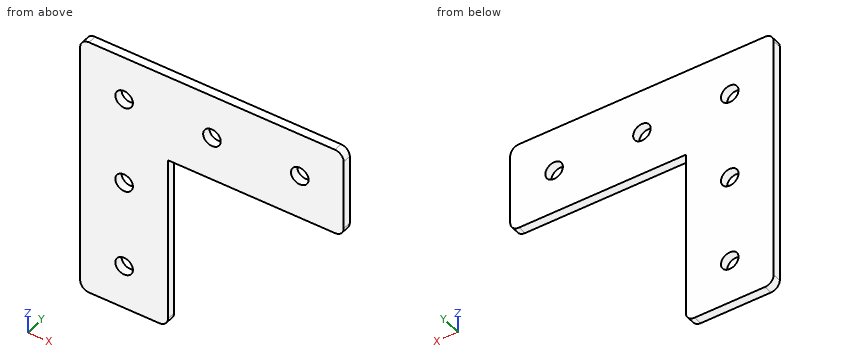
```python
from build123d import *

# Parameters (mm, degrees)
SKETCH1_R           = 2.54
BOSS_EXTRUDE1_DEPTH = 2.54
FILLET1_R           = 2.54


with BuildPart() as part:
    # Sketch1 → Boss-Extrude1 (new body)
    with BuildSketch(Plane(origin=(0, 0, 0), x_dir=(1, 0, 0), z_dir=(0, 1, 0))):
        Polygon((25.4, 76.2), (25.4, 25.4), (76.2, 25.4), (76.2, 0), (0, 0), (0, 76.2), align=None)
        with Locations((12.7, 12.7)):
            Circle(SKETCH1_R, mode=Mode.SUBTRACT)
        with Locations((38.1, 12.7)):
            Circle(SKETCH1_R, mode=Mode.SUBTRACT)
        with Locations((63.5, 12.7)):
            Circle(SKETCH1_R, mode=Mode.SUBTRACT)
        with Locations((12.7, 38.1)):
            Circle(SKETCH1_R, mode=Mode.SUBTRACT)
        with Locations((12.7, 63.5)):
            Circle(SKETCH1_R, mode=Mode.SUBTRACT)
    extrude(amount=BOSS_EXTRUDE1_DEPTH)

    # Fillet1
    fillet1_edges = [part.edges().sort_by_distance(p)[0] for p in [
        (0, 1.27, -76.2),
        (25.4, 1.27, -76.2),
        (76.2, 1.27, -25.4),
        (76.2, 1.27, 0),
        (0, 1.27, 0),
    ]]
    fillet(fillet1_edges, radius=FILLET1_R)


solid = part.part
```
The listing builds one solid part. Answer for the finished solid, in the listing's coordinates (mm). Coordinates: 2 decimals unless noted, no trailing zeros. Loops run counter-clockwise (first coordinate to the right, second up) from the corner with the lowest first, then second, coordinate; pieces in that order, holes last. Notation, with made-up numbers: (-7.75, 64) -> (19.25, 64) arc R18 cw to (19.25, 88) -> close; hole circle Ø3 at (-39.5, 79.25). An arc over 180 degrees is marked (long way). Return JSON: item names as keys, results as strings. Group by question number.
(1) Find the intervals of material crossed by probe 1 along Z at (x, y) = (12.7, 1.1); probe 2 along Z at (x, y) = (38.1, 1.9); probe 3 along X at (y, z) = (0.65, -12.7), in increasing order. Write a range as from..to.
(2) A cutting plane is placed at B-B on z = -12.7. Write down the section's boundary in (x, y).
(3) Given pin 1 Ø3 at (x, z) = (12.7, -38.1) entering from +Y; pin 2 Ø1.3 at (y, z) = (2, -42) entering from +X; pin 3 Ø6.5 at (x, z) = (12.7, -12.7) entering from -Y, each flat-ended and moving along its own axis, determine where each tip first touches the part or whether it passes through.
(4) A cutting plane is placed at D-D on y = 1.45. Write down the section's boundary in (x, z), and give its area (3 significant figures).
(5) A cutting plane is placed at A-A on x = 38.1. Write down the section's boundary in (y, z).
(6) A cutting plane is placed at C-C on x = 12.7. Write down the section's boundary in (y, z).
The answers:
{
 "1": {"probe 1": "z = -76.2..-66.04, -60.96..-40.64, -35.56..-15.24, -10.16..0", "probe 2": "z = -25.4..-15.24, -10.16..0", "probe 3": "x = 0..10.16, 15.24..35.56, 40.64..60.96, 66.04..76.2"},
 "2": {"outline": "(0, 0) -> (10.16, 0) -> (10.16, 2.54) -> (0, 2.54) -> close; (15.24, 0) -> (35.56, 0) -> (35.56, 2.54) -> (15.24, 2.54) -> close; (40.64, 0) -> (60.96, 0) -> (60.96, 2.54) -> (40.64, 2.54) -> close; (66.04, 0) -> (76.2, 0) -> (76.2, 2.54) -> (66.04, 2.54) -> close"},
 "3": {"pin 1": "passes through", "pin 2": "stops at x = 25.4", "pin 3": "stops at y = 0"},
 "4": {"outline": "(0, -73.66) arc R2.54 ccw to (2.54, -76.2) -> (22.86, -76.2) arc R2.54 ccw to (25.4, -73.66) -> (25.4, -25.4) -> (73.66, -25.4) arc R2.54 ccw to (76.2, -22.86) -> (76.2, -2.54) arc R2.54 ccw to (73.66, 0) -> (2.54, 0) arc R2.54 ccw to (0, -2.54) -> close; hole circle Ø5.08 at (12.7, -63.5); hole circle Ø5.08 at (12.7, -38.1); hole circle Ø5.08 at (12.7, -12.7); hole circle Ø5.08 at (38.1, -12.7); hole circle Ø5.08 at (63.5, -12.7)", "area": "3,120 mm^2"},
 "5": {"outline": "(0, -25.4) -> (2.54, -25.4) -> (2.54, -15.24) -> (0, -15.24) -> close; (0, -10.16) -> (2.54, -10.16) -> (2.54, 0) -> (0, 0) -> close"},
 "6": {"outline": "(0, -76.2) -> (2.54, -76.2) -> (2.54, -66.04) -> (0, -66.04) -> close; (0, -60.96) -> (2.54, -60.96) -> (2.54, -40.64) -> (0, -40.64) -> close; (0, -35.56) -> (2.54, -35.56) -> (2.54, -15.24) -> (0, -15.24) -> close; (0, -10.16) -> (2.54, -10.16) -> (2.54, 0) -> (0, 0) -> close"}
}
